Here's how the part is built. I have some questions about the finished solid (model axes, mm). A direction names the side the tool comes from. Coordinates: 2 decimals unless noted, no trailing zeros. Write each loop counter-clockwise with the first axis right and the second up, starting at its lowest first coordinate (ties: lowest second). Pieces come first, ordered by that corner, then holes.
(1) Imagine slicing it at D-D, the plane x = 19. List the corners of the cut face in (y, z) for me.
(2) Imagine slicing it at A-A, the plane y = 52.5. List the corners of the cut face in (x, z) for me (3 decimals), plus the area to 3 significant figures.
(3) For pin 1 Ø12 at (x, z) = (20, -4) entering from +Y; pin 2 Ø1 at (x, y) = (17, 80) entering from -Z, each with a flat end and sliding along its axis, tell me the tip position at first contact or that it passes through.
(4) Imagine slicing it at B-B, the plane z = -2.75. List the corners of the cut face in (x, y) for me, plus the area to 3 significant figures.
(5) Which directions (+Z, -Z, +X, -X, +Y, -Y) give clear straight access to the entire face, cutting with the end or side of a thin tool? Please do faces 1 (the flat face through (25.4, 25, -13)), 2 (the flat face through (15, 50.8, -10)).
(6) Please list where these lines run through material, in increasing order: probe 1 along Y at (x, z) = (17.25, -23.25); probe 2 along X at (y, z) = (51, -13); probe 3 along X at (y, z) = (61, -14.25).
(7) Imagine slicing it at C-C, the plane x = 14.5. List the corners of the cut face in (y, z) for me.
```python
from build123d import *

# Parameters (mm, degrees)
SKETCH1_W           = 25.4
SKETCH1_H           = 25.4
BOSS_EXTRUDE1_DEPTH = 50.8
SKETCH2_R           = 3.175
BOSS_EXTRUDE2_DEPTH = 50.8
CUT_EXTRUDE1_DEPTH  = 1.27


with BuildPart() as part:
    # Sketch1 → Boss-Extrude1 (new body)
    with BuildSketch(Plane(origin=(0, 0, 0), x_dir=(1, 0, 0), z_dir=(0, 1, 0))):
        with Locations((12.7, 12.7)):
            Rectangle(SKETCH1_W, SKETCH1_H)
    extrude(amount=BOSS_EXTRUDE1_DEPTH)

    # Sketch2 → Boss-Extrude2 (add)
    with BuildSketch(Plane(origin=(0, 50.8, 0), x_dir=(1, 0, 0), z_dir=(0, 1, 0))):
        with Locations((12.648058093, 12.7)):
            Circle(SKETCH2_R)
    extrude(amount=BOSS_EXTRUDE2_DEPTH)

    # Sketch3 → Cut-Extrude1 (cut)
    with BuildSketch(Plane.ZY):
        Polygon((-20.429638912, 24.416659376), (-20.010503295, 27.591659376), (-19.969798167, 27.591659376), (-18.658965835, 24.986531171), (-17.351313592, 27.591659376), (-17.309972446, 27.591659376), (-16.888292758, 24.416659376), (-17.174500691, 24.416659376), (-17.478517117, 26.701234697), (-18.624620883, 24.416659376), (-18.688858664, 24.416659376), (-19.839414553, 26.706322838), (-20.142794962, 24.416659376), align=None)
        Polygon((-16.237010707, 27.591659376), (-14.445985066, 27.591659376), (-14.445985066, 27.26601835), (-15.95207481, 27.26601835), (-15.95207481, 26.289095273), (-14.445985066, 26.289095273), (-14.445985066, 25.963454248), (-15.95207481, 25.963454248), (-15.95207481, 24.742300402), (-14.445985066, 24.742300402), (-14.445985066, 24.416659376), (-16.237010707, 24.416659376), align=None)
        with BuildLine():
            add(Edge.make_bspline(
                [(-12.390376092, 27.673069632), (-12.331585881, 27.671580576), (-12.216117058, 27.668655947), (-12.046413401, 27.646268474), (-11.884402136, 27.607537656), (-11.72876351, 27.555954808), (-11.581359167, 27.487144044), (-11.4410796, 27.403972516), (-11.308258579, 27.305568872), (-11.184686325, 27.192693787), (-11.071604663, 27.069881654), (-10.971976895, 26.93881955), (-10.888481386, 26.800299922), (-10.819914279, 26.654739026), (-10.766121969, 26.502466055), (-10.72900255, 26.34266921), (-10.705291514, 26.176383855), (-10.702519488, 26.062966628), (-10.701113271, 26.005431411)],
                knots=[0, 0, 0, 0, 0.000176342, 0.00034635, 0.000512345, 0.00067546, 0.000837376, 0.000999356, 0.00116396, 0.001332355, 0.001500709, 0.001664166, 0.001825381, 0.001984993, 0.002146116, 0.00230887, 0.002476442, 0.002648971, 0.002648971, 0.002648971, 0.002648971], degree=3))
            add(Edge.make_bspline(
                [(-10.701113271, 26.005431411), (-10.702519281, 25.948320013), (-10.70529069, 25.835746832), (-10.72902951, 25.670516708), (-10.76625956, 25.511684433), (-10.819414744, 25.359515162), (-10.887655, 25.213848372), (-10.971706477, 25.07506735), (-11.070713146, 24.943126598), (-11.183386504, 24.819471537), (-11.306214592, 24.706080975), (-11.437959191, 24.607275994), (-11.575657417, 24.522254824), (-11.721081224, 24.454415349), (-11.872301972, 24.400193678), (-12.030673079, 24.363225221), (-12.195452453, 24.339379117), (-12.307821149, 24.336640892), (-12.364935387, 24.33524912)],
                knots=[0, 0, 0, 0, 0.000171259, 0.000337571, 0.000499706, 0.000660019, 0.000820206, 0.000981421, 0.001145895, 0.001314289, 0.001482643, 0.001646609, 0.00180761, 0.001967222, 0.002127146, 0.002288662, 0.002454344, 0.002625603, 0.002625603, 0.002625603, 0.002625603], degree=3))
            add(Edge.make_bspline(
                [(-12.364935387, 24.33524912), (-12.422470305, 24.336654635), (-12.535886943, 24.339425279), (-12.702381254, 24.363175554), (-12.86229035, 24.400315165), (-13.01515694, 24.453391582), (-13.161066269, 24.521987213), (-13.300303701, 24.605629757), (-13.432310356, 24.704877663), (-13.555991798, 24.817514485), (-13.669157142, 24.940134393), (-13.767817433, 25.071519753), (-13.851478785, 25.209092917), (-13.919844094, 25.353235671), (-13.973968282, 25.503251194), (-14.010893367, 25.66014017), (-14.034783838, 25.82300815), (-14.037536877, 25.933899922), (-14.038933784, 25.990166988)],
                knots=[0, 0, 0, 0, 0.00017253, 0.000340102, 0.000503474, 0.000664388, 0.000824575, 0.000986335, 0.001150809, 0.001319204, 0.001487557, 0.001650632, 0.001811303, 0.001969765, 0.00212849, 0.002288769, 0.002452562, 0.00262128, 0.00262128, 0.00262128, 0.00262128], degree=3))
            add(Edge.make_bspline(
                [(-14.038933784, 25.990166988), (-14.038448793, 26.027933767), (-14.03748493, 26.102990879), (-14.025881038, 26.214448437), (-14.009042923, 26.324113534), (-13.984911188, 26.431674323), (-13.953350176, 26.536867502), (-13.916110122, 26.640418551), (-13.87062612, 26.741278072), (-13.819208675, 26.839923863), (-13.761821178, 26.934818177), (-13.698433891, 27.024516085), (-13.631273235, 27.109770275), (-13.557646442, 27.188371485), (-13.479980095, 27.262606302), (-13.397014281, 27.33133391), (-13.309255245, 27.395174044), (-13.216325372, 27.452705353), (-13.120514508, 27.504738282), (-13.021747717, 27.549389533), (-12.921366399, 27.587712746), (-12.818900396, 27.618774066), (-12.71462181, 27.643295984), (-12.608303049, 27.659994084), (-12.500028812, 27.671627572), (-12.427084258, 27.672586878), (-12.390376092, 27.673069632)],
                knots=[0, 0, 0, 0, 0.000113256, 0.000225083, 0.000335817, 0.000445988, 0.000555461, 0.000665116, 0.000775867, 0.0008871, 0.000998686, 0.001108262, 0.001216432, 0.001323994, 0.001431064, 0.001538557, 0.001646949, 0.001756368, 0.001866213, 0.001973803, 0.002081296, 0.002188332, 0.002294783, 0.002402377, 0.00251104, 0.002621117, 0.002621117, 0.002621117, 0.002621117], degree=3))
        make_face()
        with BuildLine():
            add(Edge.make_bspline(
                [(-12.376383704, 27.347428607), (-12.406514122, 27.347061313), (-12.466486908, 27.346330238), (-12.555645023, 27.336700268), (-12.643630563, 27.322975297), (-12.730461698, 27.303397775), (-12.815775118, 27.276724098), (-12.900366045, 27.24602556), (-12.983463101, 27.208632142), (-13.064791958, 27.166384046), (-13.143636348, 27.119621811), (-13.218033584, 27.067940279), (-13.288176268, 27.012551448), (-13.35389266, 26.953326052), (-13.414989795, 26.889962485), (-13.472670203, 26.823421347), (-13.524621895, 26.751800703), (-13.572233811, 26.677042691), (-13.614840352, 26.599244685), (-13.652727495, 26.519225738), (-13.683719131, 26.436333123), (-13.708994287, 26.351466137), (-13.729949115, 26.264759191), (-13.743224175, 26.175554528), (-13.752959958, 26.084300391), (-13.753649247, 26.022631138), (-13.753997887, 25.991439023)],
                knots=[0, 0, 0, 0, 9.035e-05, 0.000179837, 0.000268716, 0.000357433, 0.000446559, 0.000536708, 0.000627246, 0.000719699, 0.000811541, 0.000902048, 0.000991247, 0.001079509, 0.001167217, 0.001255174, 0.001343459, 0.001432386, 0.001520911, 0.0016094, 0.001697761, 0.001786094, 0.001874954, 0.00196509, 0.002056475, 0.002150004, 0.002150004, 0.002150004, 0.002150004], degree=3))
            add(Edge.make_bspline(
                [(-13.753997887, 25.991439023), (-13.752841405, 25.945571866), (-13.750566247, 25.855336978), (-13.730647594, 25.723104447), (-13.699966232, 25.596024359), (-13.654738478, 25.474792056), (-13.598177563, 25.358365456), (-13.52830317, 25.24777739), (-13.445518142, 25.142997968), (-13.351480514, 25.044758688), (-13.248680631, 24.955091423), (-13.139521654, 24.876384617), (-13.025173024, 24.809791033), (-12.905336548, 24.755539289), (-12.780651994, 24.712550026), (-12.65031593, 24.683087268), (-12.515196585, 24.663696677), (-12.423093776, 24.661834534), (-12.376383704, 24.660890145)],
                knots=[0, 0, 0, 0, 0.000137527, 0.000270558, 0.000400289, 0.000529072, 0.000657927, 0.000787976, 0.000920685, 0.001057889, 0.001195382, 0.001329354, 0.001461022, 0.001591668, 0.001723409, 0.001855936, 0.001992028, 0.002132069, 0.002132069, 0.002132069, 0.002132069], degree=3))
            add(Edge.make_bspline(
                [(-12.376383704, 24.660890145), (-12.344987942, 24.661321496), (-12.282720716, 24.662176993), (-12.190105492, 24.67079365), (-12.099158786, 24.684611131), (-12.01000816, 24.704505369), (-11.922754796, 24.729403906), (-11.83703451, 24.758983774), (-11.753760347, 24.795887437), (-11.67188178, 24.83666165), (-11.593508046, 24.883143793), (-11.518690956, 24.933071258), (-11.449316317, 24.988378506), (-11.383649088, 25.046723951), (-11.322301113, 25.109284013), (-11.265687249, 25.175977357), (-11.213998129, 25.247224953), (-11.166404292, 25.321869571), (-11.123947047, 25.399880457), (-11.086954578, 25.480189522), (-11.055570959, 25.562599014), (-11.030235815, 25.647227797), (-11.010382575, 25.733915138), (-10.996702934, 25.822777109), (-10.987133993, 25.913635941), (-10.986412744, 25.975089297), (-10.986049169, 26.006067429)],
                knots=[0, 0, 0, 0, 9.4165e-05, 0.000186757, 0.000278778, 0.000369977, 0.000460573, 0.00055089, 0.000641754, 0.000733627, 0.000825145, 0.000914934, 0.00100324, 0.001091077, 0.00117833, 0.001265874, 0.00135327, 0.001442197, 0.00153128, 0.001619501, 0.001707267, 0.0017956, 0.001884317, 0.001973824, 0.00206521, 0.002158103, 0.002158103, 0.002158103, 0.002158103], degree=3))
            add(Edge.make_bspline(
                [(-10.986049169, 26.006067429), (-10.986413035, 26.036833636), (-10.987134832, 26.097864076), (-10.996698363, 26.188089247), (-11.010397028, 26.276311803), (-11.030138913, 26.362185396), (-11.055584409, 26.445731915), (-11.086960059, 26.526872893), (-11.123958152, 26.605910613), (-11.166419899, 26.682649725), (-11.214149967, 26.756286809), (-11.266305459, 26.826683283), (-11.323786882, 26.892517127), (-11.384951919, 26.9554136), (-11.451328365, 27.014031257), (-11.522615546, 27.068389543), (-11.597948025, 27.119800299), (-11.677710589, 27.166178488), (-11.760028318, 27.209008542), (-11.84449598, 27.24570338), (-11.930156663, 27.276883803), (-12.016792537, 27.303478478), (-12.10513281, 27.32289862), (-12.194580569, 27.336712636), (-12.28501206, 27.346326886), (-12.345829838, 27.347060201), (-12.376383704, 27.347428607)],
                knots=[0, 0, 0, 0, 9.2258e-05, 0.00018301, 0.000271889, 0.000359986, 0.000447102, 0.00053368, 0.000620747, 0.000708715, 0.000796571, 0.000883833, 0.000971308, 0.00105856, 0.001146873, 0.001236684, 0.001327357, 0.001420293, 0.001513311, 0.001605595, 0.001696341, 0.001786684, 0.001877263, 0.001967398, 0.00205815, 0.002149772, 0.002149772, 0.002149772, 0.002149772], degree=3))
        make_face(mode=Mode.SUBTRACT)
        Polygon((-10.253356861, 27.591659376), (-9.958880699, 27.591659376), (-9.337491476, 25.263198839), (-8.413357863, 27.591659376), (-8.372016717, 27.591659376), (-7.465055579, 25.27909928), (-6.840486268, 27.591659376), (-6.549190194, 27.591659376), (-7.405269922, 24.416659376), (-7.44597505, 24.416659376), (-8.401273528, 26.84497468), (-9.368020323, 24.416659376), (-9.408725451, 24.416659376), align=None)
    extrude(amount=-CUT_EXTRUDE1_DEPTH, mode=Mode.SUBTRACT)


solid = part.part
```
Recorded:
1. outline: (0, -25.4) - (50.8, -25.4) - (50.8, 0) - (0, 0) - close
2. outline: circle Ø6.35 at (12.648, -12.7)
2. area: 31.7 mm2
3. pin 1: stops at y = 50.8
3. pin 2: passes through
4. outline: (0, 0) - (25.4, 0) - (25.4, 50.8) - (0, 50.8) - close
4. area: 1,290 mm2
5. face 1: +Z, -Z, +X, +Y, -Y
5. face 2: +Y
6. probe 1: y = 0 to 50.8
6. probe 2: x = 9.49 to 15.81
6. probe 3: x = 9.88 to 15.42
7. outline: (0, -25.4) - (50.8, -25.4) - (50.8, -15.28) - (101.6, -15.28) - (101.6, -10.12) - (50.8, -10.12) - (50.8, 0) - (0, 0) - close
